```python
from build123d import *

# Parameters (mm, degrees)
F2_DEPTH = 15
F4_DEPTH = 18
F6_D     = 3.3
F8_D     = 3.3
F9_R     = 1
F10_R    = 2.6


with BuildPart() as f2:
    # F1 (on Top) → F2 (new body)
    with BuildSketch(Plane.XY):
        Polygon((0, 3), (0, 0), (7.6, 0), (7.6, 10), (20.6, 10), (20.6, 0), (28.2, 0), (28.2, 3), (22.2, 3), (22.2, 11.6), (6, 11.6), (6, 3), align=None)
    extrude(amount=F2_DEPTH)

    # F3 (on face) → F4 (join)
    with BuildSketch(Plane.XY.offset(15)):
        Polygon((6, 0), (7.6, 0), (7.6, 10), (20.6, 10), (20.6, 0), (22.2, 0), (22.2, 3), (22.2, 11.6), (6, 11.6), (6, 3), align=None)
    extrude(amount=F4_DEPTH)

    # F6 (through all)
    with Locations(Plane(origin=(0, 3, 0), x_dir=(-1, 0, 0), z_dir=(0, 1, 0))):
        with Locations((-3.5, 7.5)):
            Hole(F6_D / 2)

    # F8 (through all)
    with Locations(Plane(origin=(0, 3, 0), x_dir=(-1, 0, 0), z_dir=(0, 1, 0))):
        with Locations((-24.7, 7.5)):
            Hole(F8_D / 2)

    # F9
    f9_edges = [f2.edges().sort_by_distance(p)[0] for p in [
        (20.6, 10, 16.5),
        (7.6, 10, 16.5),
        (28.2, 3, 7.5),
        (0, 3, 7.5),
    ]]
    fillet(f9_edges, radius=F9_R)

    # F10
    f10_edges = [f2.edges().sort_by_distance(p)[0] for p in [
        (6, 11.6, 16.5),
        (22.2, 11.6, 16.5),
    ]]
    fillet(f10_edges, radius=F10_R)


solid = f2.part
```
The model under review builds one solid part; all positions refer to its coordinate system, in mm. A direction names the side the tool comes from. Give positions to 0.01 mm unless a question says otherwise; leave off trailing zeros. Write each loop counter-clockwise with the first axis right and the second up, starting at its lowest first coordinate (ties: lowest second). Pieces come first, ordered by that corner, then holes.
(1) Consider section B-B, the plane z = 7.5. Give the boundary of the cut face in (x, y), and give its area (3 significant figures).
(2) Tool access review of faces 4 (the cylindrical face through (20.299, 9.715, 16.731)), 5 (the flat face through (3, 2, 15)), 6 (the flat face through (25.3, 3, 5.7)), 7 (the flat face through (25, 2, 15)), 8 (the flat face through (4.1, 3, 5.7)): name each direction out of +Z, -Z, +X, -X, +Y, -Y from which nothing blocks a thin tool from reaching the whole face with its end or side.
(3) To check wall thickness, follow L1, parallel to Z at x = 3.5, y = 2.1; L2, parallel to X at y = 7.25, z = 30; L3, parallel to X at y = 1.75, z = 10. State the ranges of each line that lie inside material, in increasing order.
(4) The part is to be moulded in two halves that separate along Z. For faces 1 (the flat face through (7.6, 4, 16)), 2 (the cylindrical face through (2.284, 1.479, 8.615)), 3 (the flat face through (13, 11, 0)), say which applies: released by +Z, released by -Z, zero draft, split by the parting line, or undercut.
(5) For P1, Ø4, axis at x = 3.5, z = 7.5, coming from the +Y side; P2, Ø1, axis at y = 3.5, z = 21, coming from the +X side; P3, Ø5.5, axis at x = 4.5, z = 9.5, coming from the +Y side; P4, Ø10, axis at x = 12.5, z = 5, coming from the -Y side, all flat-tipped, find the tip position at first contact; note any pin that passes through.
(6) Consider section A-A, the plane y = 8.5. Give the boundary of the cut face in (x, z).
(7) Consider section C-C, the plane x = 3.5. Give the boundary of the cut face in (y, z).
(8) Consider section D-D, the plane z = 19. Give the boundary of the cut face in (x, y), and give its area (3 significant figures).
Returned:
1. outline: (0, 0) - (1.85, 0) - (1.85, 3) - (1, 3) arc R1 ccw to (0, 2) - close; (5.15, 0) - (7.6, 0) - (7.6, 9) arc R1 cw to (8.6, 10) - (19.6, 10) arc R1 cw to (20.6, 9) - (20.6, 0) - (23.05, 0) - (23.05, 3) - (22.2, 3) - (22.2, 9) arc R2.6 ccw to (19.6, 11.6) - (8.6, 11.6) arc R2.6 ccw to (6, 9) - (6, 3) - (5.15, 3) - close; (26.35, 0) - (28.2, 0) - (28.2, 2) arc R1 ccw to (27.2, 3) - (26.35, 3) - close
1. area: 71.2 mm2
2. face 4: +Z, -Z, -Y
2. face 5: +Z, -X, +Y, -Y
2. face 6: +Z, -Z, +X, +Y
2. face 7: +Z, +X, +Y, -Y
2. face 8: +Z, -Z, -X, +Y
3. L1: z = 0 to 5.85, 9.15 to 15
3. L2: x = 6 to 7.6, 20.6 to 22.2
3. L3: x = 0 to 7.6, 20.6 to 28.2
4. face 1: zero draft
4. face 2: undercut
4. face 3: released by -Z
5. P1: stops at y = 3
5. P2: stops at x = 22.2
5. P3: stops at y = 11.22
5. P4: stops at y = 0
6. outline: (6, 0) - (7.6, 0) - (7.6, 33) - (6, 33) - close; (20.6, 0) - (22.2, 0) - (22.2, 33) - (20.6, 33) - close
7. outline: (0, 0) - (3, 0) - (3, 5.85) - (0, 5.85) - close; (0, 9.15) - (3, 9.15) - (3, 15) - (0, 15) - close
8. outline: (6, 0) - (7.6, 0) - (7.6, 9) arc R1 cw to (8.6, 10) - (19.6, 10) arc R1 cw to (20.6, 9) - (20.6, 0) - (22.2, 0) - (22.2, 9) arc R2.6 ccw to (19.6, 11.6) - (8.6, 11.6) arc R2.6 ccw to (6, 9) - close
8. area: 55.4 mm2
